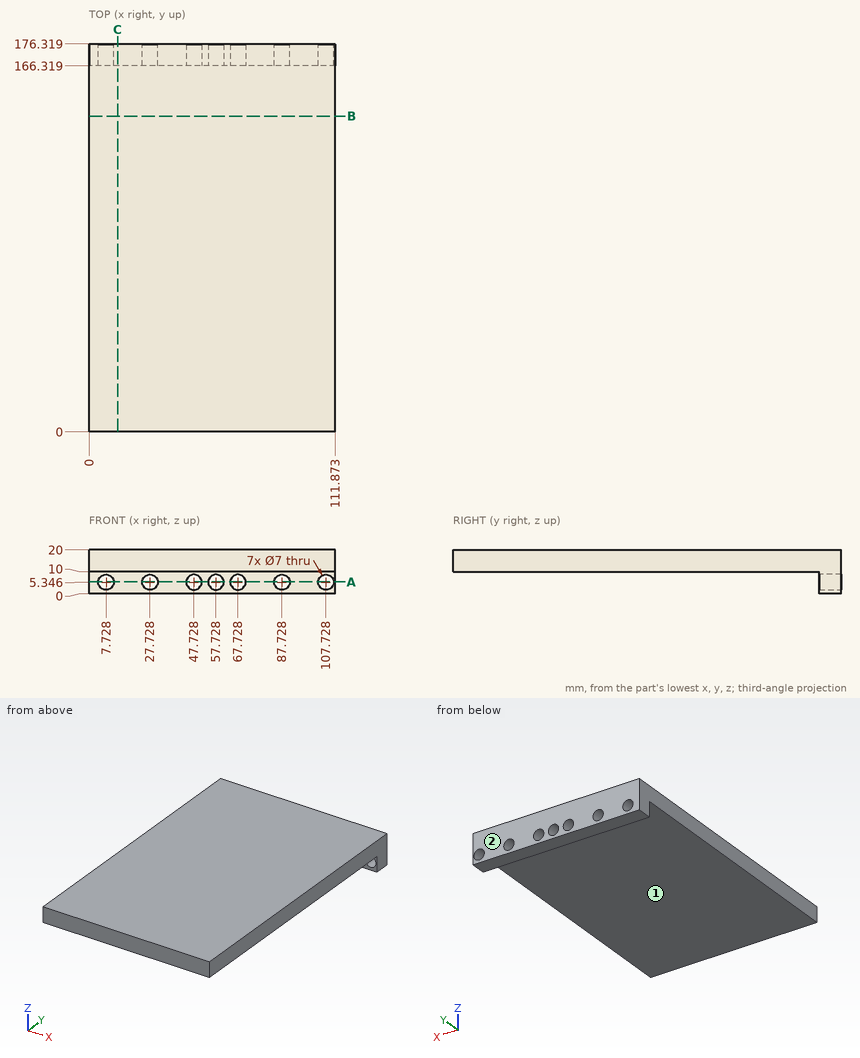
The figure shows three views and two pictorial views of one solid part (mm, origin at its lowest corner). Answer the questions. A direction names the side the tool comes from. Round coordinates to 2 decimals unless told otherwise and drop trailing zeros. Order: outer loops, then holes, each group sorted by start corner. A loop starts at its lowest first (then second) coordinate and runs counter-clockwise, first axis right, second up. Notation, with made-up numbers: (31.5, 29.5) -> (59.5, 29.5) arc R27 cw to (59.5, 61.5) -> close; hole circle Ø9 at (89, 30.25). An arc over 180 degrees is marked (long way). One line per item, written item: value.
Item 1: Straight lines are drawn through the part: L1, parallel to Z at x = 22.5, y = 81; L2, parallel to Y at x = 39.5, z = 4.75. For each, find the intervals that lie inside material, in ascending order.
Taken from the geometry:
L1: z = 10 to 20
L2: y = 166.32 to 176.32
Item 2: Find section A-A, the plane z = 5.5. State how many separate pieces and enclosed holes the cut face has, then the cut area to 3 significant figures.
Taken from the geometry:
separate pieces: 8
enclosed holes: 0
area: 629 mm2
Item 3: Find section C-C, the plane x = 13. Give the vertices of the cut face in (y, z), then the cut area to 3 significant figures.
Taken from the geometry:
outline: (0, 10) -> (166.32, 10) -> (166.32, 0) -> (176.32, 0) -> (176.32, 20) -> (0, 20) -> close
area: 1,860 mm2
Item 4: For the marked faces 1 and 2, determine the directions among +Z, -Z, +X, -X, +Y, -Y from which every point of the face is accessible in a straight line to the end or side of a thin tool.
Taken from the geometry:
face 1: -Z, +X, -X, -Y
face 2: +Z, -Z, +X, -X, +Y
Item 5: Given P1, Ø5, axis at x = 28.5, z = 7, coming from the -Y side; P2, Ø1, axis at x = 93, y = 70.5, coming from the -Z side, each flat-ended and moving along its own axis, determine where each tip first touches the part or whether it passes through.
Taken from the geometry:
P1: stops at y = 166.32
P2: stops at z = 10
Item 6: Find section B-B, the plane y = 143.5. Give the vertices of the cut face in (x, z).
Taken from the geometry:
outline: (0, 10) -> (111.87, 10) -> (111.87, 20) -> (0, 20) -> close
